from build123d import *

# Parameters (mm, degrees)
SKICA1_W                 = 20
SKICA1_H                 = 20
P_IDAT_VYSUNUT_M1_DEPTH  = 10
SKICA2_W                 = 17
SKICA2_H                 = 17
ODEBRAT_VYSUNUT_M1_DEPTH = 7.5
SKICA3_R                 = 2.65
P_IDAT_VYSUNUT_M2_DEPTH  = 7.5
ODEBRAT_VYSUNUT_M2_DEPTH = 7.5


with BuildPart() as part:
    # Skica1 → Přidat vysunutím1 (new body)
    with BuildSketch(Plane.XY):
        Rectangle(SKICA1_W, SKICA1_H)
    extrude(amount=P_IDAT_VYSUNUT_M1_DEPTH)

    # Skica2 → Odebrat vysunutím1 (cut)
    with BuildSketch(Plane(origin=(0, 0, 0), x_dir=(-1, 0, 0), z_dir=(0, 0, -1))):
        Rectangle(SKICA2_W, SKICA2_H)
    extrude(amount=-ODEBRAT_VYSUNUT_M1_DEPTH, mode=Mode.SUBTRACT)

    # Skica3 → Přidat vysunutím2 (add)
    with BuildSketch(Plane(origin=(0, 0, 7.5), x_dir=(-1, 0, 0), z_dir=(0, 0, -1))):
        with Locations(Location((0, 0, 0), (0, 0, 180))):
            Circle(SKICA3_R)
    extrude(amount=P_IDAT_VYSUNUT_M2_DEPTH)

    # Skica4 → Odebrat vysunutím2 (cut)
    with BuildSketch(Plane(origin=(0, 0, 0), x_dir=(-1, 0, 0), z_dir=(0, 0, -1))):
        Polygon((-0.585, 2.05), (0.585, 2.05), (0.585, 0.585), (2.05, 0.585), (2.05, -0.585), (0.585, -0.585), (0.585, -2.05), (-0.585, -2.05), (-0.585, -0.585), (-2.05, -0.585), (-2.05, 0.585), (-0.585, 0.585), align=None)
    extrude(amount=-ODEBRAT_VYSUNUT_M2_DEPTH, mode=Mode.SUBTRACT)


solid = part.part
Model file for the job. Use its own axes, mm. A direction names the side the tool comes from. Round coordinates to 2 decimals unless told otherwise and drop trailing zeros. Loops run counter-clockwise (first coordinate to the right, second up) from the corner with the lowest first, then second, coordinate; pieces in that order, holes last. Notation, with made-up numbers: (-6.5, 86.5) -> (24.5, 86.5) arc R8 ccw to (24.5, 96.5) -> close; hole circle Ø3 at (55, 80.5). An arc over 180 degrees is marked (long way). Answer as CSV lines item,"result". Start each with the question number.
1) Slice it at A-A (z = 1.75). List the corners of the cut face in (x, y) (3 decimals).
2) Mould opens along Y. For faces 1 (the face through (0, 10, 5)), 2 (the face through (-1, -0.585, 4)), 3 (the face through (0, -10, 5)) say: +Y half, -Y half, draft (parallel to the pull), parting line (faces both ways), or undercut.
3) Tool access for faces 4 (the face through (0, 0, 10)), 5 (the face through (2.05, 0, 4)): list every direction of +Z, -Z, +X, -X, +Y, -Y with a clear straight run to the whole face (end or side of a thin tool).
4) Slice it at D-D (x = 0). List the corners of the cut face in (y, z), plus the area to 3 significant figures.
5) Probe line 1 along X through (y, z) = (8.25, 4.5); line 2 along Y through (x, z) = (0, 4.75). List the from-to ranges inside material, lowest first.
6) Slice it at B-B (x = 6.25). List the corners of the cut face in (y, z).
Filled in:
1,outline,"(-10, -10) -> (10, -10) -> (10, 10) -> (-10, 10) -> close; circle Ø5.3 at (0, 0); hole (-8.5, -8.5) -> (8.5, -8.5) -> (8.5, 8.5) -> (-8.5, 8.5) -> close; hole (-2.05, -0.585) -> (-0.585, -0.585) -> (-0.585, -2.05) -> (0.585, -2.05) -> (0.585, -0.585) -> (2.05, -0.585) -> (2.05, 0.585) -> (0.585, 0.585) -> (0.585, 2.05) -> (-0.585, 2.05) -> (-0.585, 0.585) -> (-2.05, 0.585) -> close"
2,face 1,"+Y half"
2,face 2,"undercut"
2,face 3,"-Y half"
3,face 4,"+Z, +X, -X, +Y, -Y"
3,face 5,"-Z"
4,outline,"(-10, 0) -> (-8.5, 0) -> (-8.5, 7.5) -> (-2.65, 7.5) -> (-2.65, 0) -> (-2.05, 0) -> (-2.05, 7.5) -> (2.05, 7.5) -> (2.05, 0) -> (2.65, 0) -> (2.65, 7.5) -> (8.5, 7.5) -> (8.5, 0) -> (10, 0) -> (10, 10) -> (-10, 10) -> close"
4,area,"81.5 mm2"
5,line 1,"x = -10 to -8.5, 8.5 to 10"
5,line 2,"y = -10 to -8.5, -2.65 to -2.05, 2.05 to 2.65, 8.5 to 10"
6,outline,"(-10, 0) -> (-8.5, 0) -> (-8.5, 7.5) -> (8.5, 7.5) -> (8.5, 0) -> (10, 0) -> (10, 10) -> (-10, 10) -> close"
